Could you check a few things on this drawing? It's one solid part, dimensions in mm from its lowest x, y, z. A direction names the side the tool comes from. Give positions to 0.01 mm unless a question says otherwise; leave off trailing zeros. Loops run counter-clockwise (first coordinate to the right, second up) from the corner with the lowest first, then second, coordinate; pieces in that order, holes last. Notation, with made-up numbers: (40, 6.5) - (50, 6.5) arc R7 ccw to (50, 17.5) - close; hole circle Ø10 at (4.25, 76). An arc over 180 degrees is marked (long way). Put each result on its own line as item: value. Start each with the question number.
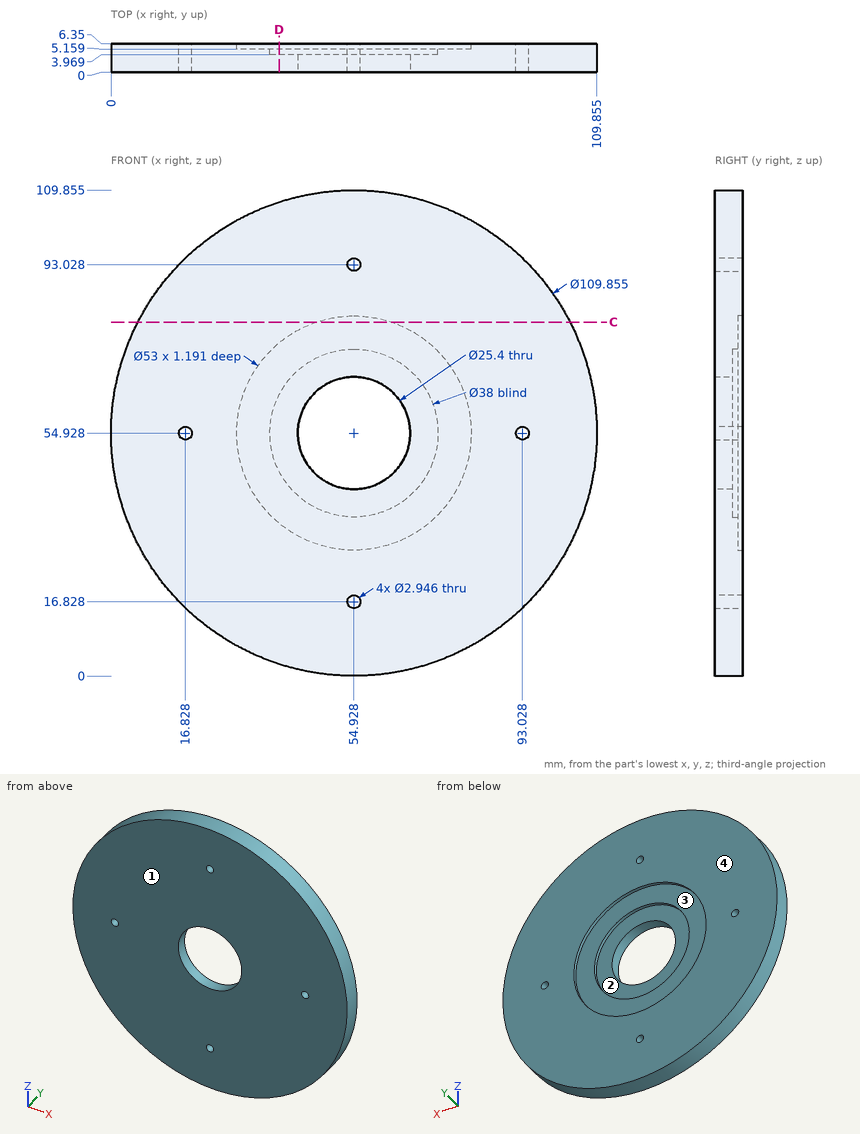
1) I need wall thicknesses on line 1 (Y direction, x = 47.5, z = 34); line 2 (X direction, y = 4.25, z = 67.5) (1 decimal); line 3 (X direction, y = 5.5, z = 48.5) (1 decimal). Which ranges of each line are inside material? Lowest first, please.
2) Suppose I cut it at D-D on x = 38. Please give me the cut outline in (y, z).
3) Suppose I cut it at C-C on z = 80. Please give me the cut outline in (x, y).
4) Which directions (+Z, -Z, +X, -X, +Y, -Y) give clear straight access to the entire face, cutting with the end or side of a thin tool? Please do the marked faces 3 and 4.
5) Thinking about a two-plate mould opening in Z: for the marked faces 1 and 2, which applies, pulls with the +Z half, pulls with the -Z half, needs draft (parallel to the pull), parting line crosses it, or undercut?
6) I'm going to push flat-ended pins straight in: P1, Ø1.5, axis at x = 84.5, y = 4, coming from the -Z side; P2, Ø3, axis at y = 4, z = 67, coming from the -X side; P3, Ø16, axis at x = 43.5, z = 63.5, coming from the +Y side. Where does each tip first touch, or does it pass through?
Ans:
1. line 1: y = 0 to 5.16
1. line 2: x = 1.5 to 40.7, 69.2 to 108.4
1. line 3: x = 0.4 to 29.2, 80.6 to 109.5
2. outline: (0, 2.67) - (6.35, 2.67) - (6.35, 34.54) - (5.16, 34.54) - (5.16, 46.3) - (3.97, 46.3) - (3.97, 63.56) - (5.16, 63.56) - (5.16, 75.32) - (6.35, 75.32) - (6.35, 107.18) - (0, 107.18) - close
3. outline: (6.06, 0) - (103.8, 0) - (103.8, 6.35) - (63.51, 6.35) - (63.51, 5.16) - (46.35, 5.16) - (46.35, 6.35) - (6.06, 6.35) - close
4. face 3: +Y
4. face 4: +Z, -Z, +X, -X, +Y
5. face 1: needs draft
5. face 2: undercut
6. P1: stops at z = 8.17
6. P2: stops at x = 1.03
6. P3: stops at y = 5.16
